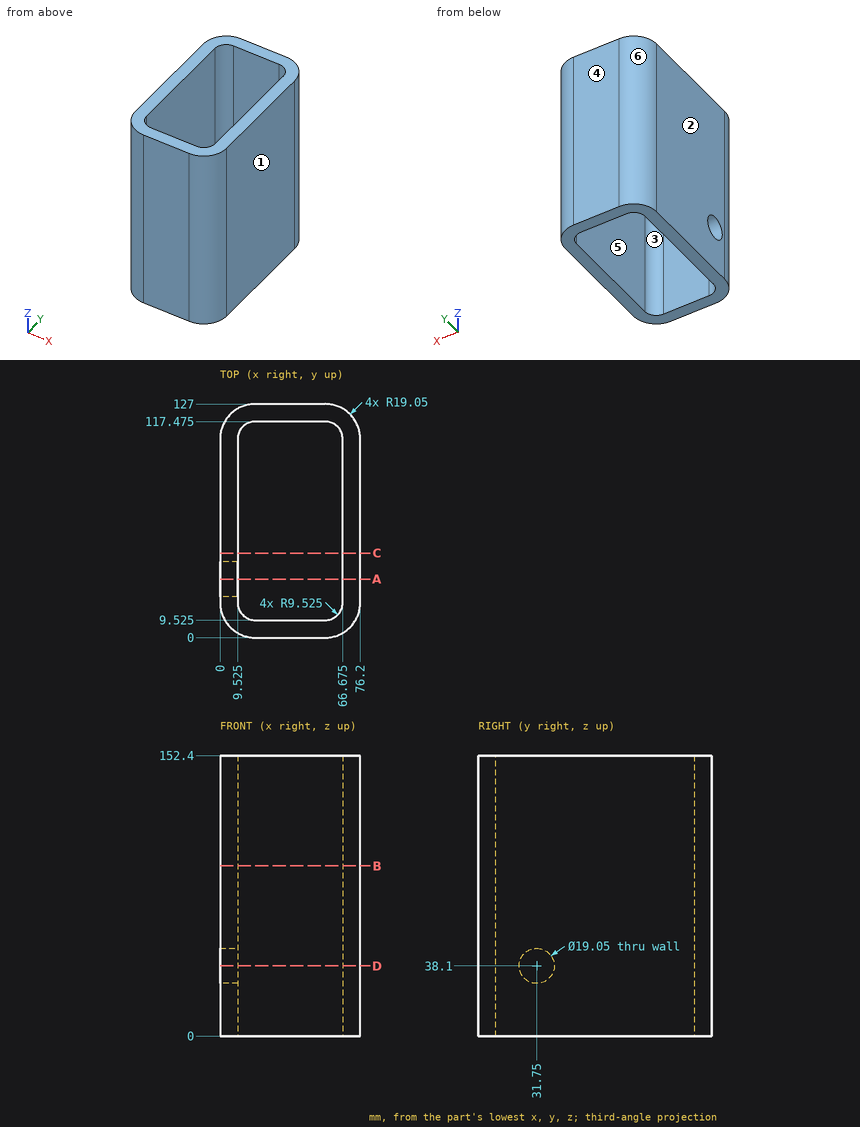
Input: dimensioned drawing with shaded views. Units: mm. Origin: part minimum x, y, z. A direction names the side the tool comes from. Coordinates: 2 decimals unless noted, no trailing zeros. Loops run counter-clockwise (first coordinate to the right, second up) from the corner with the lowest first, then second, coordinate; pieces in that order, holes last. Notation, with made-up numbers: M 6.5,24 L 60.5,24 A23 cw 60.5,55 Z; hole C -12,3.5 d10. An arc over 180 degrees is marked long. One line per item, written item: value. Start each with the question number.
1) Material intervals for L1, parallel to Z at x = 5, y = 31; L2, parallel to X at y = 27.5, z = 57 (3 decimals); L3, parallel to Y at x = 20, z = 110.5 (3 decimals), sorted ascending. Write a range as from..to.
2) Pin query (flat end, axial travel): P1, Ø4, axis at y = 114, z = 87.5, coming from the +X side; P2, Ø11.5, axis at y = 31.75, z = 38.1, coming from the -X side (3 decimals). Return the tip coordinate at first contact, or that it passes through.
3) Cut plane A-A (y = 31.75). Return loops of the section in (x, z) (3 decimals), then the cut area to 3 significant figures.
4) Draft query along X for the marked faces 1, 2, 3 and 4. Return one class per face: released by +X, released by -X, zero draft, split by the parting line, or undercut.
5) Cut plane D-D (z = 38.1). Return loops of the section in (x, y) (3 decimals), then the cut area to 3 significant figures.
6) Cut plane C-C (y = 46). Return loops of the section in (x, z) (3 decimals).
7) Reachability of the marked faces 5 and 6 from +Z, -Z, +X, -X, +Y, -Y: full face, straight path, thin tool, end or side. Return the list, or none.
8) Cut plane B-B (z = 92.5). Return loops of the section in (x, y) (3 decimals).
Evaluation:
1. L1: 0..28.6, 47.6..152.4
1. L2: 0..9.525, 66.675..76.2
1. L3: 0..9.525, 117.475..127
2. P1: x = 75.76
2. P2: x = 66.675
3. outline: M 0,0 L 9.525,0 L 9.525,28.575 L 0,28.575 Z; M 0,47.625 L 9.525,47.625 L 9.525,152.4 L 0,152.4 Z; M 66.675,0 L 76.2,0 L 76.2,152.4 L 66.675,152.4 Z
3. area: 2,720 mm^2
4. face 1: released by +X
4. face 2: released by -X
4. face 3: undercut
4. face 4: zero draft
5. outline: M 0,19.05 A19.05 ccw 19.05,0 L 57.15,0 A19.05 ccw 76.2,19.05 L 76.2,107.95 A19.05 ccw 57.15,127 L 19.05,127 A19.05 ccw 0,107.95 L 0,41.275 L 9.525,41.275 L 9.525,107.95 A9.525 cw 19.05,117.475 L 57.15,117.475 A9.525 cw 66.675,107.95 L 66.675,19.05 A9.525 cw 57.15,9.525 L 19.05,9.525 A9.525 cw 9.525,19.05 L 9.525,22.225 L 0,22.225 Z
5. area: 3,090 mm^2
6. outline: M 0,0 L 9.525,0 L 9.525,152.4 L 0,152.4 Z; M 66.675,0 L 76.2,0 L 76.2,152.4 L 66.675,152.4 Z
7. face 5: +Z, -Z
7. face 6: +Z, -Z, -X, +Y
8. outline: M 0,19.05 A19.05 ccw 19.05,0 L 57.15,0 A19.05 ccw 76.2,19.05 L 76.2,107.95 A19.05 ccw 57.15,127 L 19.05,127 A19.05 ccw 0,107.95 Z; hole M 9.525,19.05 A9.525 ccw 19.05,9.525 L 57.15,9.525 A9.525 ccw 66.675,19.05 L 66.675,107.95 A9.525 ccw 57.15,117.475 L 19.05,117.475 A9.525 ccw 9.525,107.95 Z
